```python
from build123d import *

# Parameters (mm, degrees)
F0_W          = 65.024
F0_H          = 84.074
F1_DEPTH      = 35.052
F1_DEPTH_BACK = 35.052
F3_DEPTH      = 63.5
F4_W          = 77.3881527235
F4_H          = 70.5238262352
F5_DEPTH      = 38.1
F7_DEPTH      = 25.4
F9_DEPTH      = 38.1
F10_T1_DEPTH  = 70.104


# Not quite as in the source:
# - a fillet or chamfer that OpenCascade refuses, or shapes differently, is made with other operations: its cross-section is extruded or revolved along the edge and cut away or added


with BuildPart() as f1:
    # F0 (on Right) → F1 (new body, two sides)
    with BuildSketch(Plane.YZ) as f1_sk:
        Rectangle(F0_W, F0_H)
    extrude(amount=F1_DEPTH)
    extrude(f1_sk.sketch, amount=-F1_DEPTH_BACK)

    # F2 (on Front) → F3 (cut, symmetric)
    with BuildSketch(Plane.XZ):
        Polygon((-11.176, -16.637), (-11.176, -3.937), (-78.232, -3.937), (-78.232, -87.8102174824), (-11.176, -87.8102174824), (-11.176, -21.463), (-5.588, -21.463), (-5.588, -16.637), align=None)
        Polygon((75.6774835046, -3.937), (11.176, -3.937), (11.176, -16.637), (5.588, -16.637), (5.588, -21.463), (11.176, -21.463), (11.176, -87.8102174824), (75.6774835046, -87.8102174824), align=None)
    extrude(amount=F3_DEPTH, both=True, mode=Mode.SUBTRACT)

    # F4 (on Right) → F5 (cut, symmetric)
    with BuildSketch(Plane.YZ):
        with Locations((45.8060763618, 28.2769131176)):
            Rectangle(F4_W, F4_H)
    extrude(amount=F5_DEPTH, both=True, mode=Mode.SUBTRACT)

    # F6 (on face) → F7 (cut, symmetric)
    with BuildSketch(Plane.YZ.offset(11.176)):
        Polygon((32.512, -21.463), (32.512, -42.037), (58.1510797716, -47.1596371092), (55.1210400309, 2.9251785083), (22.86, 2.9251785083), (28.0953935412, -21.463), align=None)
        Polygon((28.0953935412, -21.463), (32.512, -42.037), (32.512, -21.463), align=None)
    extrude(amount=F7_DEPTH, both=True, mode=Mode.SUBTRACT)

    # F8 (on Right) → F9 (cut, symmetric)
    with BuildSketch(Plane.YZ):
        with BuildLine():
            ThreePointArc((-27.8538692881, 15.113), (-17.5873761822, 39.8985068942), (7.1981307119, 50.165))
            Line((7.1981307119, 50.165), (-30.8227688074, 66.0536216443))
            Line((-30.8227688074, 66.0536216443), (-47.4338419735, 15.113))
            Line((-47.4338419735, 15.113), (-27.8538692881, 15.113))
        make_face()
    extrude(amount=F9_DEPTH, both=True, mode=Mode.SUBTRACT)

    # F10: fillet of radius 6.35 on 1 edges, made by hand

    # F10_s2 → F10_t1 (join)
    with BuildSketch(Plane.YZ.offset(-35.052)):
        with BuildLine():
            ThreePointArc((-32.512, 15.113), (-29.1481831988, 16.9504285484), (-27.454542127, 20.3888856242))
            ThreePointArc((-27.454542127, 20.3888856242), (-27.7538949257, 17.7584882017), (-27.8538692881, 15.113))
            Line((-27.8538692881, 15.113), (-32.512, 15.113))
        make_face()
    extrude(amount=F10_T1_DEPTH)


solid = f1.part
```
For this review, take the finished solid that the model builds, in its own axes (mm). A direction names the side the tool comes from. Coordinates: 2 decimals unless noted, no trailing zeros. Write each loop counter-clockwise with the first axis right and the second up, starting at its lowest first coordinate (ties: lowest second). Pieces come first, ordered by that corner, then holes. Notation, with made-up numbers: (-24, 80.5) - (13, 80.5) arc R16 ccw to (13, 106.5) - close; hole circle Ø8 at (-30.75, 39). An arc over 180 degrees is marked (long way). Answer in a Markdown table with one row per item. Add a question column.
Q1. For probe 1 along X at (y, z) = (6, -33.5); probe 2 along Y at (x, z) = (-4.5, 12); probe 3 along Z at (x, y) = (-20.5, -2.5), list the stretches that pass through material, from the lowest coordinate up.
Q2. We need section C-C, the plane x = -1. State the section outline as (y, z) points (3 decimals), and give its area (3 significant figures).
Q3. We need section A-A, the plane x = -9. State the section outline as (y, z) points (3 decimals).
Q4. We need section B-B, the plane y = -9.5. State the section outline as (x, z) points, and give its area (3 significant figures).
Q5. Draft analysis for pull direction Z (two halves, no side actions). For faces 4 (the flat face through (-8, -2, -16.637)), 5 (the flat face through (8, -3, -21.463)), 6 (the flat face through (0, -32.512, -8)), 7 (the cylindrical face through (-0.49, -29.19, 16.91)), state which applies: +Z half, -Z half, draft (parallel to the pull), parting line (faces both ways), or undercut.
Q6. For P1, Ø2, axis at y = -21, z = -29.5, coming from the +X side; P2, Ø5.5, axis at y = 12, z = -18.5, coming from the -X side; P3, Ø3, axis at x = 24, y = -23, coming from the +Z side; P4, Ø5, axis at x = -14, z = -8.5, coming from the +Y side, all flat-tipped, find the tip position at first contact; note any pin that passes through.
Q7. We need section D-D, the plane y = 18.5. State the section outline as (x, z) points (3 decimals), and give its area (3 significant figures).
Q8. Tool access review of faces 1 (the flat face through (11.176, -3, -10)), 2 (the flat face through (-11.176, -2, -10)), 3 (the flat face through (-5.588, -2, -19)): name each direction out of +Z, -Z, +X, -X, +Y, -Y from which nothing blocks a thin tool from reaching the whole face with its end or side.
Answer list:
| question | item | result |
|---|---|---|
| 1 | probe 1 | x = -11.18 to 11.18 |
| 1 | probe 2 | y = -32.51 to 7.11 |
| 1 | probe 3 | z = -3.94 to 42.04 |
| 2 | outline | (-32.512, -42.037) - (32.512, -42.037) - (24.987, -6.985) - (7.112, -6.985) - (7.112, 42.037) - (-15.246, 42.037) arc R35.052 ccw to (-27.455, 20.389) arc R6.35 cw to (-32.512, 15.113) - close |
| 2 | area | 3,870 mm2 |
| 3 | outline | (-32.512, -42.037) - (32.512, -42.037) - (28.095, -21.463) - (-32.512, -21.463) - close; (-32.512, -16.637) - (27.059, -16.637) - (24.987, -6.985) - (7.112, -6.985) - (7.112, 42.037) - (-15.246, 42.037) arc R35.052 ccw to (-27.455, 20.389) arc R6.35 cw to (-32.512, 15.113) - close |
| 4 | outline | (-35.05, -3.94) - (-11.18, -3.94) - (-11.18, -16.64) - (-5.59, -16.64) - (-5.59, -21.46) - (-11.18, -21.46) - (-11.18, -42.04) - (11.18, -42.04) - (11.18, -21.46) - (5.59, -21.46) - (5.59, -16.64) - (11.18, -16.64) - (11.18, -3.94) - (35.05, -3.94) - (35.05, 42.04) - (-35.05, 42.04) - close |
| 4 | area | 4,020 mm2 |
| 5 | face 4 | undercut |
| 5 | face 5 | undercut |
| 5 | face 6 | draft |
| 5 | face 7 | +Z half |
| 6 | P1 | stops at x = 11.18 |
| 6 | P2 | stops at x = -11.18 |
| 6 | P3 | stops at z = 35.24 |
| 6 | P4 | passes through |
| 7 | outline | (-11.176, -42.037) - (11.176, -42.037) - (11.176, -21.463) - (5.588, -21.463) - (5.588, -16.637) - (11.176, -16.637) - (11.176, -6.985) - (-11.176, -6.985) - (-11.176, -16.637) - (-5.588, -16.637) - (-5.588, -21.463) - (-11.176, -21.463) - close |
| 7 | area | 730 mm2 |
| 8 | face 1 | -Z, +X, +Y, -Y |
| 8 | face 2 | -Z, -X, +Y, -Y |
| 8 | face 3 | -X, +Y, -Y |
